from build123d import *

# Parameters (mm, degrees)
BOSS_EXTRUDE1_DEPTH = 50
SKETCH2_W           = 4.47
SKETCH2_H           = 5
CUT_EXTRUDE2_DEPTH  = 10
CHAMFER1_SIZE       = 0.3
FILLET1_R           = 0.75


with BuildPart() as part:
    # Sketch1 → Boss-Extrude1 (new body)
    with BuildSketch(Plane.XY):
        with BuildLine():
            ThreePointArc((2.35, 1.86480562), (0, 3), (-2.35, 1.86480562))
            Line((-2.35, 1.86480562), (2.35, 1.86480562))
        make_face()
        with BuildLine():
            Line((2.35, 1.86480562), (-2.35, 1.86480562))
            ThreePointArc((-2.35, 1.86480562), (-0.987420883, -2.832843095), (3, 0))
            ThreePointArc((3, 0), (2.832843095, 0.987420883), (2.35, 1.86480562))
        make_face()
    extrude(amount=BOSS_EXTRUDE1_DEPTH)

    # Sketch2 → Cut-Extrude2 (cut)
    with BuildSketch(Plane.XY.offset(50)):
        with Locations((0, 4.501193394)):
            Rectangle(SKETCH2_W, SKETCH2_H)
    extrude(amount=-CUT_EXTRUDE2_DEPTH, mode=Mode.SUBTRACT)

    # Chamfer1
    chamfer1_edges = [part.edges().sort_by_distance(p)[0] for p in [
        (-0.089200091, -2.998673597, 50),
        (0, 2.001193394, 50),
    ]]
    chamfer(chamfer1_edges, length=CHAMFER1_SIZE)

    # Fillet1
    fillet1_edges = [part.edges().sort_by_distance(p)[0] for p in [
        (0, 2.001193394, 40),
    ]]
    fillet(fillet1_edges, radius=FILLET1_R)


solid = part.part
The listing builds one solid part. Answer for the finished solid, in the listing's coordinates (mm). A direction names the side the tool comes from. Give positions to 0.01 mm unless a question says otherwise; leave off trailing zeros. Write each loop counter-clockwise with the first axis right and the second up, starting at its lowest first coordinate (ties: lowest second). Pieces come first, ordered by that corner, then holes.
1) Find the intervals of material crossed by L1, parallel to Z at x = -0.5, y = 2.75; L2, parallel to Y at x = -2, z = 40; L3, parallel to Y at x = 0.25, z = 29, in increasing order.
2) Given P1, Ø1.5, axis at y = -1.5, z = 11, coming from the +X side; P2, Ø3.5, axis at x = 1, z = 46, coming from the +Y side; P3, Ø2, axis at x = -1.5, z = 37.5, coming from the +Y side, each flat-ended and moving along its own axis, determine where each tip first touches the part or whether it passes through.
3) A tool of negligible diameter and unlimited length cuts with its end or side. For faces 1 (the face through (0, 2.001, 45)), 2 (the face through (0, 0, 0)), from which of +Z, -Z, +X, -X, +Y, -Y can it reach the whole face along a straight path? Write none if from no direction.
4) Section A-A (x = 0) is taken. Write down the section's boundary in (y, z), and give its area (3 significant figures).
5) Section B-B (z = 15) is taken. Write down the section's boundary in (x, y), and give its area (3 significant figures).
Response:
1. L1: z = 0 to 40
1. L2: y = -2.24 to 2.24
1. L3: y = -2.99 to 2.99
2. P1: stops at x = 2.9
2. P2: stops at y = 2
2. P3: stops at y = 2.96
3. face 1: +Z, +X, -X, +Y
3. face 2: -Z, +X, -X, +Y, -Y
4. outline: (-3, 0) - (3, 0) - (3, 40) - (2.75, 40) arc R0.75 cw to (2, 40.75) - (2, 49.7) - (1.7, 50) - (-2.7, 50) - (-3, 49.7) - close
4. area: 290 mm2
5. outline: circle Ø6 at (0, 0)
5. area: 28.3 mm2
